from build123d import *

# Parameters (mm, degrees)
F0_W     = 574.675
F0_H     = 1828.8
F1_DEPTH = 17.4625
F2_R     = 254
F3_R     = 254
F4_R     = 63.5
F5_DEPTH = 63.5
F6_R     = 63.49999


# Not quite as in the source:
# - a fillet or chamfer is up to 0.001 mm smaller than in the source, because OpenCascade refuses the exact size


with BuildPart() as f1:
    # F0 (on Front) → F1 (new body)
    with BuildSketch(Plane.XZ):
        with Locations((-1034.1491804612, -4.0362142026)):
            Rectangle(F0_W, F0_H)
    extrude(amount=F1_DEPTH)

    # F2
    f2_edges = [f1.edges().sort_by_distance(p)[0] for p in [
        (-1321.48668, -8.73125, 910.363786),
    ]]
    fillet(f2_edges, radius=F2_R)

    # F3
    f3_edges = [f1.edges().sort_by_distance(p)[0] for p in [
        (-746.81168, -8.73125, 910.363786),
    ]]
    fillet(f3_edges, radius=F3_R)

    # F4 (on face) → F5 (join)
    with BuildSketch(Plane.XZ.offset(17.4625)):
        with Locations((-1034.1491804612, 656.3637857974)):
            Circle(F4_R)
    extrude(amount=F5_DEPTH)

    # F6 (radius 63.5 in the source; OpenCascade refuses exactly that, so slightly less here)
    f6_edges = [f1.edges().sort_by_distance(p)[0] for p in [
        (-1097.64918, -80.9625, 656.363786),
    ]]
    fillet(f6_edges, radius=F6_R)


solid = f1.part
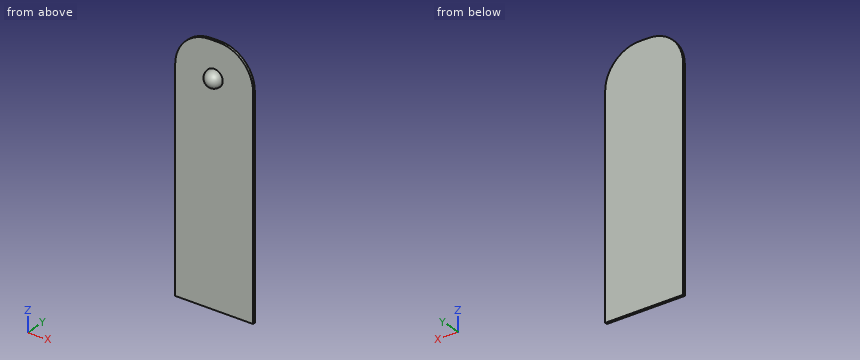
Design review of the part built by this model. Coordinates are the model's own, in mm. Give positions to 0.01 mm unless a question says otherwise; leave off trailing zeros. Loops run counter-clockwise (first coordinate to the right, second up) from the corner with the lowest first, then second, coordinate; pieces in that order, holes last. Notation, with made-up numbers: M 46,65.25 L 63,65.25 A26 ccw 63,83.25 Z; hole C -29.5,0.5 d1. An arc over 180 degrees is marked long. One line per question, with ' | ' between items. Start each with the question number.
1. To check wall thickness, follow L1, parallel to Y at x = -1244.5, z = -527; L2, parallel to Z at x = -1178.5, y = -15.5. State the ranges of each line that lie inside material, in increasing order.
2. Insertion check: P1, Ø1, axis at x = -870, y = -17.5, coming from the -Z side. The pin has a flat end and moves straight along its axis. Give the tip position at first contact, or say it passes through.
3. Add section A-A (z = -739.5). Write out the cut boundary in (x, y), plus the area to 3 significant figures.
4. Add section B-B (x = -1281). Write out the cut boundary in (y, z), plus the area to 3 significant figures.
Worked out:
1) L1: y = -17.46 to 0 | L2: z = -918.44 to 884.82
2) P1: stops at z = -918.44
3) outline: M -1321.49,-17.46 L -746.81,-17.46 L -746.81,0 L -1321.49,0 Z | area: 10,000 mm²
4) outline: M -17.46,-918.44 L 0,-918.44 L 0,793.94 L -17.46,793.94 Z | area: 29,900 mm²
